```python
from build123d import *

# Parameters (mm, degrees)
SKETCH_1_R               = 10
EXTRUDE_1_DEPTH          = 2
SKETCH_3_R               = 3
CUT_EXTRUDE_1_DEPTH      = 15.282856857
EXTRUDE_START            = 1
SKETCH_4_R               = 5
SKETCH_4_R_2             = 3
EXTRUDE_2_DEPTH          = 1
SKETCH_5_R               = 1
CUT_EXTRUDE_2_DEPTH      = 15.456832295
PATTERN_CIRCULAR_1_COUNT = 8


with BuildPart() as part:
    # 草图1 → 凸台-拉伸1 (new body)
    with BuildSketch(Plane(origin=(0, 0, 0), x_dir=(0, 0, -1), z_dir=(1, 0, 0))):
        Circle(SKETCH_1_R)
    extrude(amount=EXTRUDE_1_DEPTH)

    # 草图3 → 切除-拉伸1 (cut, through all)
    with BuildSketch(Plane(origin=(2, 0, 0), x_dir=(0, 0, -1), z_dir=(1, 0, 0))):
        Circle(SKETCH_3_R)
    extrude(amount=-CUT_EXTRUDE_1_DEPTH, mode=Mode.SUBTRACT)

    # 草图4 → 凸台-拉伸2 (add)
    with BuildSketch(Plane(origin=(2, 0, 0), x_dir=(0, 0, -1), z_dir=(1, 0, 0)).offset(EXTRUDE_START)):
        Circle(SKETCH_4_R)
        Circle(SKETCH_4_R_2, mode=Mode.SUBTRACT)
    extrude(amount=-EXTRUDE_2_DEPTH)

    # 草图5 → 切除-拉伸2 (cut, through all)
    with BuildSketch(Plane.ZY):
        with Locations((0, 7)):
            Circle(SKETCH_5_R)
    cut_extrude_2 = extrude(amount=-CUT_EXTRUDE_2_DEPTH, mode=Mode.SUBTRACT)

    # 阵列(圆周)1: 切除-拉伸2 ×8 about axis
    pattern_circular_1_axis = Axis((0, 0, 0), (1, 0, 0))
    for i in range(1, PATTERN_CIRCULAR_1_COUNT):
        add(cut_extrude_2.rotate(pattern_circular_1_axis, i * 360 / PATTERN_CIRCULAR_1_COUNT), mode=Mode.SUBTRACT)


solid = part.part
```
Part model, mm, in its own coordinate system. Round coordinates to 2 decimals unless told otherwise and drop trailing zeros. Loops run counter-clockwise (first coordinate to the right, second up) from the corner with the lowest first, then second, coordinate; pieces in that order, holes last. Notation, with made-up numbers: (82, 53.25) -> (93, 53.25) arc R30 cw to (93, 84.25) -> close; hole circle Ø6 at (1.5, 10.25). An arc over 180 degrees is marked (long way). Use one line per item in the form item = value. Start each with the question number.
Item 1: Drill centre lines: line 1 along Y through (x, z) = (1.2, 0); line 2 along X through (y, z) = (-5.5, -1.5); line 3 along Z through (x, y) = (0.4, 4.5). Where is each one in solid material? Low to high.
Item 2: Band-saw the part on A-A (y = 0). List the corners of the cut face in (x, z), plus the area to 3 significant figures.
Item 3: Band-saw the part on B-B (x = 2.65). List the corners of the cut face in (y, z).
Item 4: Drop flat-ended pins along their axis: pin 1 Ø2 at (y, z) = (7.5, -6.5) entering from -X; pin 2 Ø2.5 at (y, z) = (0, 7) entering from +X; pin 3 Ø1 at (x, z) = (1.5, 5.5) entering from +Y; pin 4 Ø1.5 at (x, z) = (1.5, -7.5) entering from +Y. Give the stop position or say it passes through.
Item 5: Two-plate mould, pull along Z, no slides. Class faces 1 (the cylindrical face through (1, 0, -8)), 2 (the flat face through (2, -2, 5)), 3 (the cylindrical face through (2.51, -4.88, 1.08)): released by +Z, released by -Z, zero draft, split by the parting line, or undercut.
Item 6: Band-saw the part on C-C (y = 7). List the corners of the cut face in (x, z).
Data:
q1.line_1 = -10 to -8, -6 to -3, 3 to 6, 8 to 10
q1.line_2 = 0 to 2
q1.line_3 = -8.93 to -5.84, -4.06 to 4.06, 5.84 to 8.93
q2.outline = (0, -10) -> (2, -10) -> (2, -8) -> (0, -8) -> close; (0, -6) -> (2, -6) -> (2, -5) -> (3, -5) -> (3, -3) -> (0, -3) -> close; (0, 3) -> (3, 3) -> (3, 5) -> (2, 5) -> (2, 6) -> (0, 6) -> close; (0, 8) -> (2, 8) -> (2, 10) -> (0, 10) -> close
q2.area = 24.0 mm^2
q3.outline = circle Ø10 at (0, 0); hole circle Ø6 at (0, 0)
q4.pin_1 = 0
q4.pin_2 = 2
q4.pin_3 = 8.66
q4.pin_4 = 7.38
q5.face_1 = undercut
q5.face_2 = zero draft
q5.face_3 = split by the parting line
q6.outline = (0, -7.14) -> (2, -7.14) -> (2, -1) -> (0, -1) -> close; (0, 1) -> (2, 1) -> (2, 7.14) -> (0, 7.14) -> close
